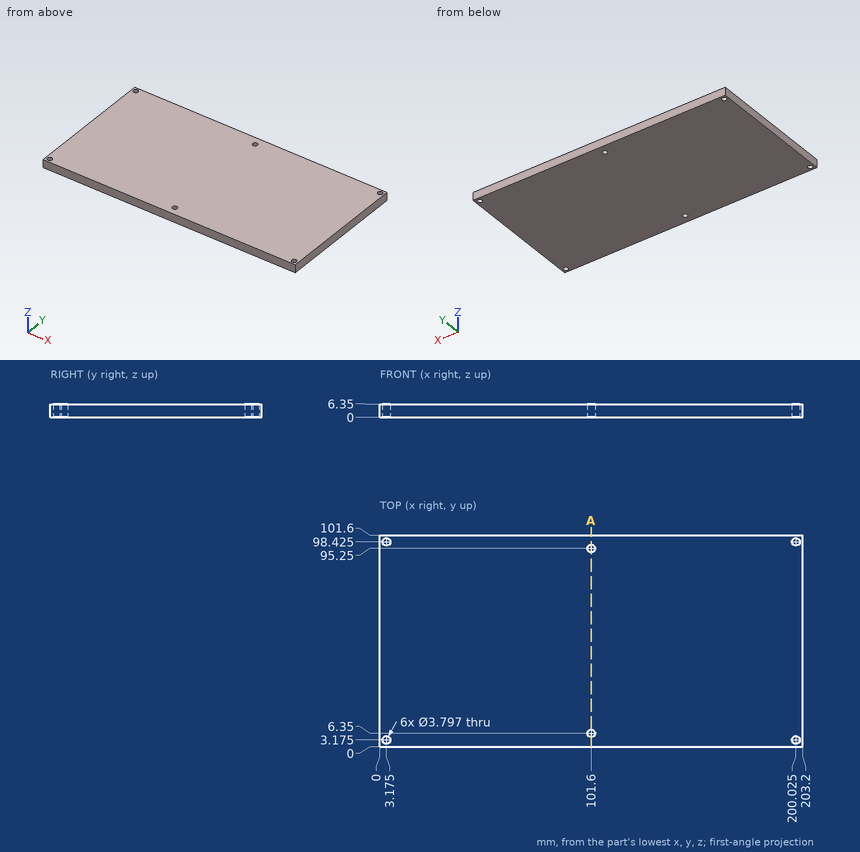
Source: three-view drawing plus pictorial views. Frame: mm from the lowest corner of the part. Give positions to 0.01 mm unless a question says otherwise; leave off trailing zeros. Order: outer loops, then holes, each group sorted by start corner. A loop starts at its lowest first (then second) coordinate and runs counter-clockwise, first axis right, second up. Notation, with made-up numbers: (52.5, 56) - (90.5, 56) arc R19 cw to (90.5, 85) - close; hole circle Ø8 at (30, -16). An arc over 180 degrees is marked (long way). Answer as a JSON object with one key per item and string values. Group by question number.
Q1. First-contact query: pin 1 Ø3 at (x, y) = (3.175, 3.175) entering from -Z. Flat tip, straight axial feed; report the tip coordinate or a pass-through.
Q2. Cut plane A-A, the plane x = 101.6. Output: boundary loops of the cut face in (y, z).
Q3. Line query: probe 1 along X at (y, z) = (95.25, 1.5); probe 2 along Y at (x, z) = (103, 3.5); probe 3 along Y at (x, z) = (101, 3). Output: solid intervals per line, ascending.
Results:
{
 "1": {"pin 1": "through"},
 "2": {"outline": "(0, 0) - (4.45, 0) - (4.45, 6.35) - (0, 6.35) - close; (8.25, 0) - (93.35, 0) - (93.35, 6.35) - (8.25, 6.35) - close; (97.15, 0) - (101.6, 0) - (101.6, 6.35) - (97.15, 6.35) - close"},
 "3": {"probe 1": "0 to 99.7, 103.5 to 203.2", "probe 2": "0 to 5.07, 7.63 to 93.97, 96.53 to 101.6", "probe 3": "0 to 4.55, 8.15 to 93.45, 97.05 to 101.6"}
}
